The drawing under review shows one solid part. Ordinate dimensions are in mm from its lowest x, y, z. Give positions to 0.01 mm unless a question says otherwise; leave off trailing zeros. Loops run counter-clockwise (first coordinate to the right, second up) from the corner with the lowest first, then second, coordinate; pieces in that order, holes last. Notation, with made-up numbers: (-28, -23) - (8, -23) arc R25 ccw to (8, 13) - close; hole circle Ø6 at (44.25, 15.5). An arc over 180 degrees is marked (long way). Put each result on its own line as item: value. Start each with the question number.
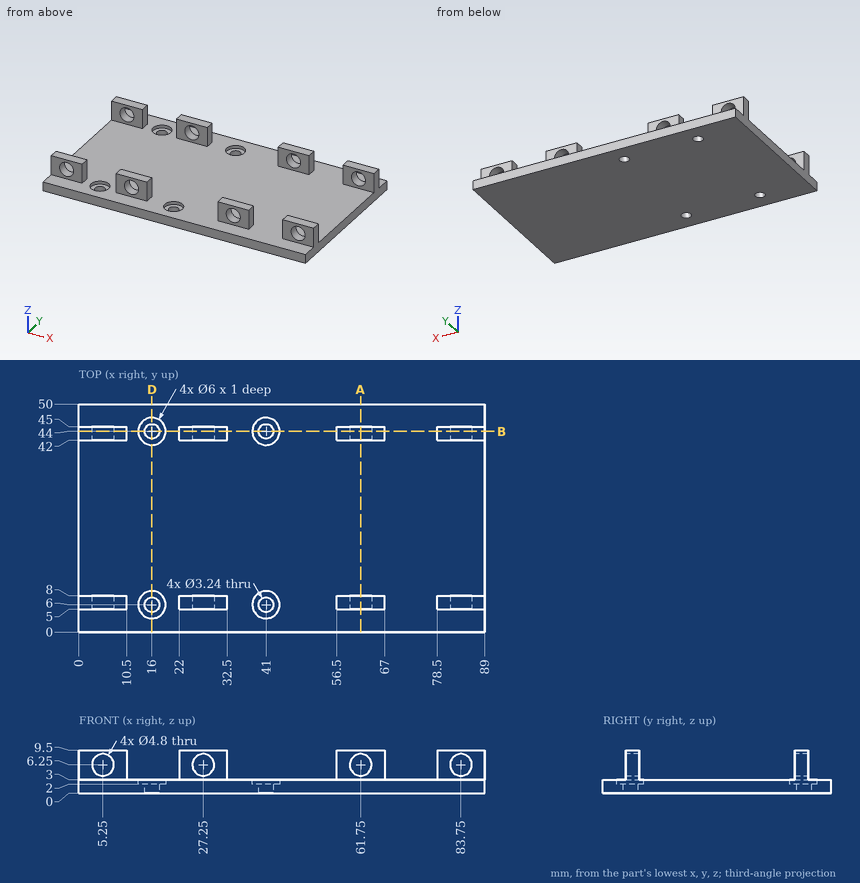
Item 1: For P1, Ø5, axis at y = 8.5, z = 4, coming from the -X side; P2, Ø3, axis at x = 29.5, y = 13.5, coming from the +Z side; P3, Ø5, axis at x = 3.5, z = 6.5, coming from the -Y side; P4, Ø3, axis at x = 63.5, z = 7, coming from the +Y side, all flat-tipped, find the tip position at first contact; note any pin that passes through.
Item 2: For L1, parallel to Z at x = 41.5, y = 10.5; L2, parallel to Z at x = 5, y = 43; L3, parallel to Y at x = 24, z = 3.25, list the stretches that pass through material, from the lowest coordinate up. Write a range as from..to.
Item 3: Consider section B-B (y = 44). Count the separate pieces of the cut face and the enclosed holes in it, plus the area to 3 significant figures.
Item 4: Consider section A-A (x = 61.75). State the section outline as (y, z) points, plus the area to 3 significant figures.
Item 5: Consider section D-D (x = 16). State the section outline as (y, z) points.
Geometry says:
1. P1: stops at x = 0
1. P2: stops at z = 3
1. P3: stops at y = 5
1. P4: stops at y = 45
2. L1: z = 0..3
2. L2: z = 0..3.86, 8.64..9.5
2. L3: y = 5..8, 42..45
3. separate pieces: 3
3. enclosed holes: 4
3. area: 443 mm2
4. outline: (0, 0) - (50, 0) - (50, 3) - (45, 3) - (45, 3.85) - (42, 3.85) - (42, 3) - (8, 3) - (8, 3.85) - (5, 3.85) - (5, 3) - (0, 3) - close; (5, 8.65) - (8, 8.65) - (8, 9.5) - (5, 9.5) - close; (42, 8.65) - (45, 8.65) - (45, 9.5) - (42, 9.5) - close
4. area: 160 mm2
5. outline: (0, 0) - (4.38, 0) - (4.38, 2) - (3, 2) - (3, 3) - (0, 3) - close; (7.62, 0) - (42.38, 0) - (42.38, 2) - (41, 2) - (41, 3) - (9, 3) - (9, 2) - (7.62, 2) - close; (45.62, 0) - (50, 0) - (50, 3) - (47, 3) - (47, 2) - (45.62, 2) - close
